Geometry check sheet. Reference: the model listing, model coordinates, mm. Round coordinates to 2 decimals unless told otherwise and drop trailing zeros. Loops run counter-clockwise (first coordinate to the right, second up) from the corner with the lowest first, then second, coordinate; pieces in that order, holes last. Notation, with made-up numbers: (28.5, -38) - (49.5, -38) arc R31 ccw to (49.5, -10) - close; hole circle Ø4 at (60, 86.25). An arc over 180 degrees is marked (long way). Write item = value, one per line.
```python
from build123d import *

# Parameters (mm, degrees)
F0_W     = 25.4
F0_H     = 50.8
F0_W_2   = 50.8
F0_H_2   = 25.4
F0_W_3   = 508
F0_H_3   = 508
F1_DEPTH = 50.8
F2_DEPTH = 25.4
F3_DEPTH = 25.4
F4_DEPTH = 25.4
F5_DEPTH = 25.4


with BuildPart() as f1:
    # F0 (on Top) → F1 (new body)
    with BuildSketch(Plane.XY):
        with Locations((307.4446349591, -113.3660624364)):
            Rectangle(F0_W, F0_H)
        with Locations((-289.4553650409, -151.4660624364)):
            Rectangle(F0_W_2, F0_H_2)
        with Locations((307.4446349591, 483.5339375636)):
            Rectangle(F0_W, F0_H_2)
        with Locations((-289.4553650409, -113.3660624364)):
            Rectangle(F0_W_2, F0_H)
        with Locations((307.4446349591, -151.4660624364)):
            Rectangle(F0_W, F0_H_2)
        with Locations((-327.5553650409, -151.4660624364)):
            Rectangle(F0_W, F0_H_2)
        with Locations((269.3446349591, -113.3660624364)):
            Rectangle(F0_W_2, F0_H)
        with Locations((-10.0553650409, -151.4660624364)):
            Rectangle(F0_W_3, F0_H_2)
        with Locations((269.3446349591, -151.4660624364)):
            Rectangle(F0_W_2, F0_H_2)
        with Locations((-10.0553650409, 483.5339375636)):
            Rectangle(F0_W_3, F0_H_2)
        with Locations((269.3446349591, 483.5339375636)):
            Rectangle(F0_W_2, F0_H_2)
        with Locations((-327.5553650409, -113.3660624364)):
            Rectangle(F0_W, F0_H)
        with Locations((-327.5553650409, 166.0339375636)):
            Rectangle(F0_W, F0_H_3)
        with Locations((269.3446349591, 166.0339375636)):
            Rectangle(F0_W_2, F0_H_3)
        with Locations((307.4446349591, 166.0339375636)):
            Rectangle(F0_W, F0_H_3)
        with Locations((307.4446349591, 445.4339375636)):
            Rectangle(F0_W, F0_H)
        with Locations((269.3446349591, 445.4339375636)):
            Rectangle(F0_W_2, F0_H)
        with Locations((-10.0553650409, 166.0339375636)):
            Rectangle(F0_W_3, F0_H_3)
        with Locations((-10.0553650409, -113.3660624364)):
            Rectangle(F0_W_3, F0_H)
        with Locations((-289.4553650409, 166.0339375636)):
            Rectangle(F0_W_2, F0_H_3)
        with Locations((-10.0553650409, 445.4339375636)):
            Rectangle(F0_W_3, F0_H)
        with Locations((-289.4553650409, 445.4339375636)):
            Rectangle(F0_W_2, F0_H)
        with Locations((-327.5553650409, 445.4339375636)):
            Rectangle(F0_W, F0_H)
        with Locations((-327.5553650409, 483.5339375636)):
            Rectangle(F0_W, F0_H_2)
        with Locations((-289.4553650409, 483.5339375636)):
            Rectangle(F0_W_2, F0_H_2)
    extrude(amount=F1_DEPTH)

    # F0 (on Top) → F2 (cut)
    with BuildSketch(Plane.XY):
        with Locations((269.3446349591, -113.3660624364)):
            Rectangle(F0_W_2, F0_H)
    extrude(amount=F2_DEPTH, mode=Mode.SUBTRACT)

    # F0 (on Top) → F3 (cut)
    with BuildSketch(Plane.XY):
        with Locations((269.3446349591, 445.4339375636)):
            Rectangle(F0_W_2, F0_H)
    extrude(amount=F3_DEPTH, mode=Mode.SUBTRACT)

    # F0 (on Top) → F4 (cut)
    with BuildSketch(Plane.XY):
        with Locations((-289.4553650409, 445.4339375636)):
            Rectangle(F0_W_2, F0_H)
    extrude(amount=F4_DEPTH, mode=Mode.SUBTRACT)

    # F0 (on Top) → F5 (cut)
    with BuildSketch(Plane.XY):
        with Locations((-289.4553650409, -113.3660624364)):
            Rectangle(F0_W_2, F0_H)
    extrude(amount=F5_DEPTH, mode=Mode.SUBTRACT)


solid = f1.part
```
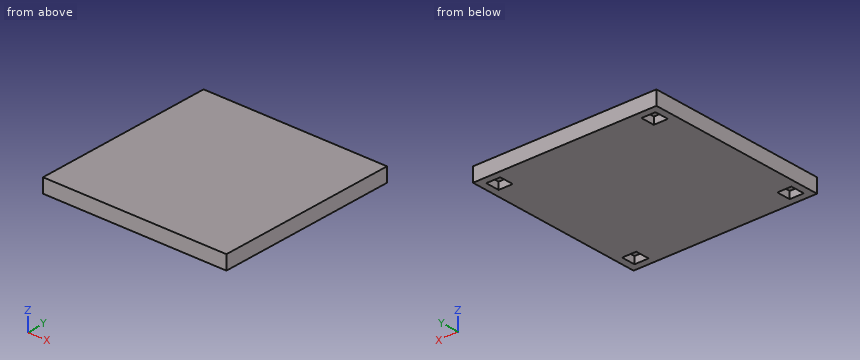
(1) Scan lines: L1, parallel to Y at x = 272, z = 15; L2, parallel to X at y = 463.5, z = 8. Record each from-to range of solid material in increasing order. Write a range as [from, to].
Answers follow:
L1 = [-164.17, -138.77], [-87.97, 420.03], [470.83, 496.23]
L2 = [-340.26, -314.86], [-264.06, 243.94], [294.74, 320.14]
(2) Gauge pin test, flat end, axial feed: pin 1 (15 mm diameter, centred on x = 281.5, y = 450.5, fed in from -Z). Record the tip position at first contact, or that the pin passes through.
Answers follow:
pin_1 = 25.4
(3) Section check A-A (z = 17.5). Enter the section's corners in (x, y), then the cut area to 3 significant figures.
Answers follow:
outline = (-340.26, -164.17) - (320.14, -164.17) - (320.14, 496.23) - (-340.26, 496.23) - close; hole (-314.86, -138.77) - (-264.06, -138.77) - (-264.06, -87.97) - (-314.86, -87.97) - close; hole (-314.86, 420.03) - (-264.06, 420.03) - (-264.06, 470.83) - (-314.86, 470.83) - close; hole (243.94, -138.77) - (294.74, -138.77) - (294.74, -87.97) - (243.94, -87.97) - close; hole (243.94, 420.03) - (294.74, 420.03) - (294.74, 470.83) - (243.94, 470.83) - close
area = 426,000 mm²
